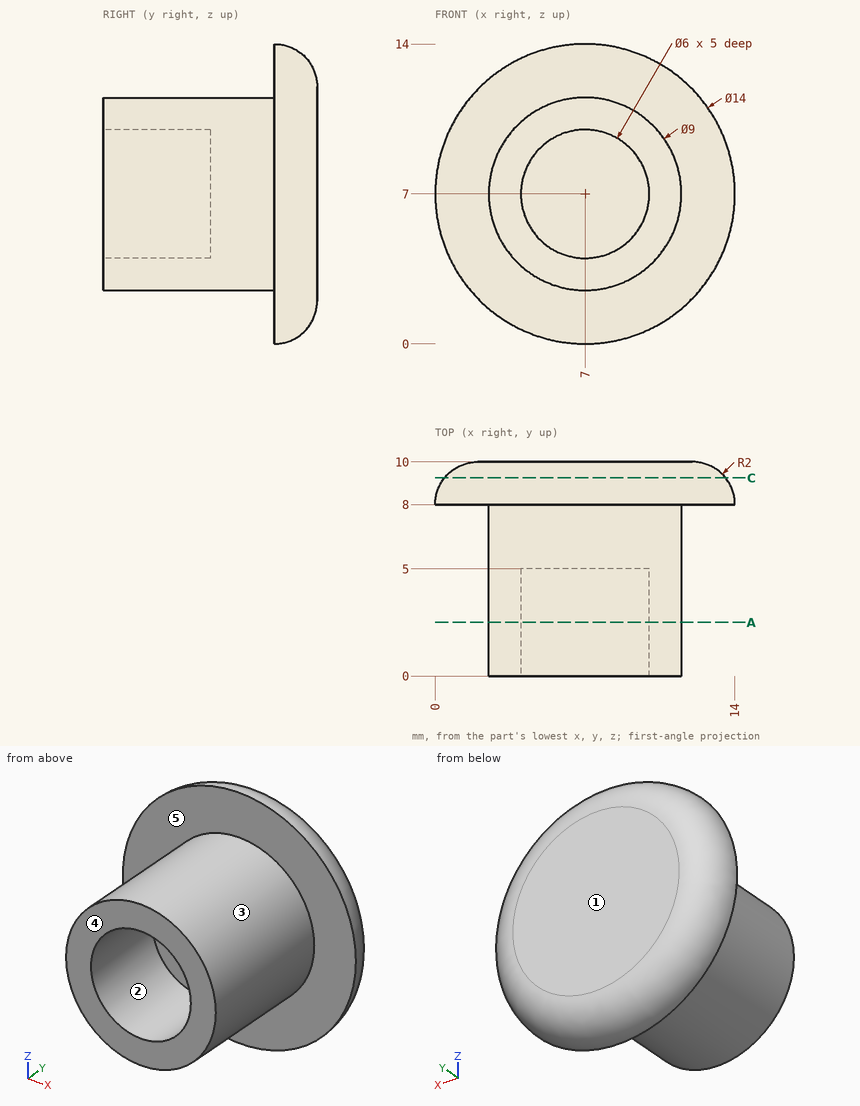
Answer from the drawing. Dimensions are ordinates in mm from the lowest x, y and z of the part. A direction names the side the tool comes from. Give positions to 0.01 mm unless a question says otherwise; leave off trailing zeros. Write each loop counter-clockwise with the first axis right and the second up, starting at its lowest first coordinate (ties: lowest second). Pieces come first, ordered by that corner, then holes. Notation, with made-up numbers: (80, -13) - (135, -13) arc R30 cw to (135, 24) - close; hole circle Ø9 at (-24.5, 76). An arc over 180 degrees is marked (long way). One line per item, written item: value. Start each with the question number.
1. For a pull along Z with two mould halves and no side action, classify the marked faces 1, 2 and 3 as +Z half, -Z half, draft (parallel to the pull), parting line (faces both ways), or undercut.
2. For the marked faces 4 and 5, determine the directions among +Z, -Z, +X, -X, +Y, -Y from which every point of the face is accessible in a straight line to the end or side of a thin tool.
3. Find section C-C (y = 9.25). Write down the section's boundary in (x, z).
4. Given pin 1 (3 mm diameter, centred on x = 8.5, y = 3.5, fed in from +Z); pin 2 (2 mm diameter, centred on x = 3, y = 5.5, fed in from -Z); pin 3 (2 mm diameter, centred on x = 7, z = 7.5, fed in from -Y), each flat-ended and moving along its own axis, determine where each tip first touches the part or whether it passes through.
5. Find section A-A (y = 2.5). Write down the section's boundary in (x, z), then the cut area to 3 significant figures.
6. Consider probe 1 along Z at (x, y) = (7, 2.05); probe 2 along Z at (x, y) = (5.5, 3.25); probe 3 along Y at (x, z) = (10.75, 10.5). Determine where each line is inside the solid, lowest interval first.
Geometry results:
1. face 1: draft
1. face 2: undercut
1. face 3: parting line
2. face 4: +Z, -Z, +X, -X, -Y
2. face 5: -Y
3. outline: circle Ø13.12 at (7, 7)
4. pin 1: z = 11.5
4. pin 2: z = 3.65
4. pin 3: y = 5
5. outline: circle Ø9 at (7, 7); hole circle Ø6 at (7, 7)
5. area: 35.3 mm2
6. probe 1: 2.5 to 4, 10 to 11.5
6. probe 2: 2.76 to 4.4, 9.6 to 11.24
6. probe 3: 8 to 10
